Geometry check sheet. Reference: the model listing, model coordinates, mm. Face numbers are marked on the shaded views. A direction names the side the tool comes from. Give positions to 0.01 mm unless a question says otherwise; leave off trailing zeros. Write each loop counter-clockwise with the first axis right and the second up, starting at its lowest first coordinate (ties: lowest second). Pieces come first, ordered by that corner, then holes. Notation, with made-up numbers: (-26.75, 2) -> (1.25, 2) arc R17 ccw to (1.25, 29) -> close; hole circle Ø11 at (-9, 13). An arc over 180 degrees is marked (long way). Use a Markdown table: item, result. Add a question column.
from build123d import *

# Parameters (mm, degrees)
F0_W     = 60
F0_H     = 60
F1_DEPTH = 45
F2_T     = -2
F3_W     = 3.4
F3_H     = 6.9295717942
F4_DEPTH = 64.2
F5_W     = 3.4
F5_H     = 10.5797095255
F6_DEPTH = 63.5
F8_DEPTH = 25


# Not quite as in the source:
# - a feature names something its author has since deleted; it is built from what else it names


with BuildPart() as f1:
    # F0 (on Top) → F1 (new body)
    with BuildSketch(Plane.XY):
        Rectangle(F0_W, F0_H)
    extrude(amount=F1_DEPTH)

    # F2
    f2_openings = [f1.faces().sort_by_distance(p)[0] for p in [
        (0, 0, 45),
    ]]
    offset(amount=F2_T, openings=f2_openings)

    # F3 (on face) → F4 (cut)
    with BuildSketch(Plane.XZ.offset(30)):
        Polygon((-20.4337567297, 35), (-6, 10), (-4, 10), (-4, 16.9295717942), (-14.4337567297, 35), align=None)
        with Locations((-1.9, 13.4647858971)):
            Rectangle(F3_W, F3_H)
        with Locations((1.9, 13.4647858971)):
            Rectangle(F3_W, F3_H)
        Polygon((4, 16.9295717942), (4, 10), (6, 10), (20.4337567297, 35), (14.4337567297, 35), align=None)
    extrude(amount=-F4_DEPTH, mode=Mode.SUBTRACT)

    # F5 (on face) → F6 (cut)
    with BuildSketch(Plane.YZ.offset(30)):
        Polygon((-20.4337567297, 35), (-6, 10), (-4, 10), (-4, 20.5797095255), (-14.4337567297, 35), align=None)
        with Locations((-1.9, 15.2898547627)):
            Rectangle(F5_W, F5_H)
        with Locations((1.9, 15.2898547627)):
            Rectangle(F5_W, F5_H)
        Polygon((4, 20.5797095255), (4, 10), (6, 10), (20.4337567297, 35), (14.4337567297, 35), align=None)
    extrude(amount=-F6_DEPTH, mode=Mode.SUBTRACT)

    # F7 (on face) → F8 (cut)
    with BuildSketch(Plane(origin=(0, 0, 0), x_dir=(1, 0, 0), z_dir=(0, 0, -1))):
        with BuildLine():
            Line((0.9656854249, 0.4), (9.9919967974, 0.4))
            ThreePointArc((9.9919967974, 0.4), (9.2387953251, 3.8268343237), (7.3482514055, 6.7825659806))
            Line((7.3482514055, 6.7825659806), (0.9656854249, 0.4))
        make_face()
        with BuildLine():
            ThreePointArc((7.3482514055, -6.7825659806), (9.2387953251, -3.8268343237), (9.9919967974, -0.4))
            Line((9.9919967974, -0.4), (0.9656854249, -0.4))
            Line((0.9656854249, -0.4), (7.3482514055, -6.7825659806))
        make_face()
        with BuildLine():
            Line((0.4, 0.9656854249), (6.7825659806, 7.3482514055))
            ThreePointArc((6.7825659806, 7.3482514055), (3.8268343237, 9.2387953251), (0.4, 9.9919967974))
            Line((0.4, 9.9919967974), (0.4, 0.9656854249))
        make_face()
        with BuildLine():
            ThreePointArc((0.4, -9.9919967974), (3.8268343237, -9.2387953251), (6.7825659806, -7.3482514055))
            Line((6.7825659806, -7.3482514055), (0.4, -0.9656854249))
            Line((0.4, -0.9656854249), (0.4, -9.9919967974))
        make_face()
        with BuildLine():
            Line((-6.7825659806, 7.3482514055), (-0.4, 0.9656854249))
            Line((-0.4, 0.9656854249), (-0.4, 9.9919967974))
            ThreePointArc((-0.4, 9.9919967974), (-3.8268343237, 9.2387953251), (-6.7825659806, 7.3482514055))
        make_face()
        with BuildLine():
            Line((-0.4, -9.9919967974), (-0.4, -0.9656854249))
            Line((-0.4, -0.9656854249), (-6.7825659806, -7.3482514055))
            ThreePointArc((-6.7825659806, -7.3482514055), (-3.8268343237, -9.2387953251), (-0.4, -9.9919967974))
        make_face()
        with BuildLine():
            Line((-7.3482514055, -6.7825659806), (-0.9656854249, -0.4))
            Line((-0.9656854249, -0.4), (-9.9919967974, -0.4))
            ThreePointArc((-9.9919967974, -0.4), (-9.2387953251, -3.8268343237), (-7.3482514055, -6.7825659806))
        make_face()
        with BuildLine():
            Line((-9.9919967974, 0.4), (-0.9656854249, 0.4))
            Line((-0.9656854249, 0.4), (-7.3482514055, 6.7825659806))
            ThreePointArc((-7.3482514055, 6.7825659806), (-9.2387953251, 3.8268343237), (-9.9919967974, 0.4))
        make_face()
    extrude(amount=-F8_DEPTH, mode=Mode.SUBTRACT)


solid = f1.part
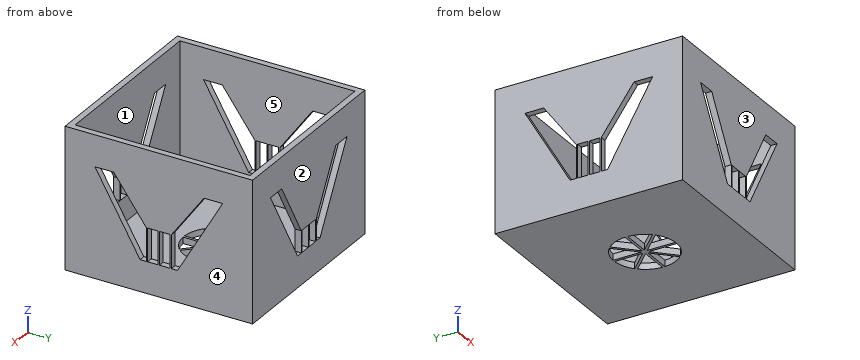
1) Sectioned sample at A-A, the plane z = 7.5. Enter the section's corners in (x, y).
2) Gauge pin test, flat end, axial feed: P1, Ø1, axis at x = -20.5, y = -7.5, coming from the +Z side. Record the tip position at first contact, or that the pin passes through.
3) Material ranges on probe 1 along X at (y, z) = (21, 38); probe 2 along Z at (x, y) = (2, 27), recorded low to high. Write a range as [from, to].
4) Sectioned sample at D-D, the plane x = -21.5. Enter the section's corners in (y, z), and give its area (3 significant figures).
5) Sectioned sample at B-B, the plane x = -11. Enter the section's corners in (y, z), and give its area (3 significant figures).
6) Sectioned sample at C-C, the plane y = -19.5. Enter the section's corners in (x, z), and give its area (3 significant figures).
7) Draft check along Y on the marked faces 3, 4 and 5. Enter one of: +Y half, -Y half, draft (parallel to the pull), parting line (faces both ways), or undercut.
8) Tool access check on the marked faces 1 and 2. Record the directions out of +Z, -Z, +X, -X, +Y, -Y that give a thin tool (end or side, any length) a straight path to the whole face; none if there is none.
Check values:
| question | item | result |
|---|---|---|
| 1 | outline | (-30, -30) -> (30, -30) -> (30, 30) -> (-30, 30) -> close; hole (-28, -28) -> (28, -28) -> (28, 28) -> (-28, 28) -> close |
| 2 | P1 | z = 2 |
| 3 | probe 1 | [-30, -28], [28, 30] |
| 3 | probe 2 | [0, 2] |
| 4 | outline | (-30, 0) -> (30, 0) -> (30, 45) -> (28, 45) -> (28, 2) -> (-28, 2) -> (-28, 45) -> (-30, 45) -> close |
| 4 | area | 292 mm² |
| 5 | outline | (-30, 0) -> (30, 0) -> (30, 18.66) -> (28, 18.66) -> (28, 2) -> (-28, 2) -> (-28, 18.66) -> (-30, 18.66) -> close; (-30, 29.05) -> (-28, 29.05) -> (-28, 45) -> (-30, 45) -> close; (28, 29.05) -> (30, 29.05) -> (30, 45) -> (28, 45) -> close |
| 5 | area | 250 mm² |
| 6 | outline | (-30, 0) -> (30, 0) -> (30, 33.38) -> (28, 33.38) -> (28, 2) -> (-28, 2) -> (-28, 33.38) -> (-30, 33.38) -> close; (-30, 35) -> (-28, 35) -> (-28, 45) -> (-30, 45) -> close; (28, 35) -> (30, 35) -> (30, 45) -> (28, 45) -> close |
| 6 | area | 286 mm² |
| 7 | face 3 | -Y half |
| 7 | face 4 | draft |
| 7 | face 5 | undercut |
| 8 | face 1 | +Z |
| 8 | face 2 | +Z, -Z, +X, -X, +Y |
